```python
from build123d import *

# Parameters (mm, degrees)
F0_W     = 60
F0_H     = 50
F1_DEPTH = 3
F2_W     = 5
F2_H     = 25
F3_DEPTH = 30
F4_R     = 12.49999
F5_R     = 3
F6_DEPTH = 50
F7_R     = 2.5
F8_DEPTH = 25


# Not quite as in the source:
# - a fillet or chamfer is up to 0.001 mm smaller than in the source, because OpenCascade refuses the exact size


with BuildPart() as f1:
    # F0 (on Top) → F1 (new body)
    with BuildSketch(Plane.XY):
        Rectangle(F0_W, F0_H)
    extrude(amount=F1_DEPTH)

    # F2 (on face) → F3 (join)
    with BuildSketch(Plane.XY.offset(3)):
        with Locations((-11.5, 0)):
            Rectangle(F2_W, F2_H)
        with Locations((11.5, 0)):
            Rectangle(F2_W, F2_H)
    extrude(amount=F3_DEPTH)

    # F4 (radius 12.5 in the source; OpenCascade refuses exactly that, so slightly less here)
    f4_edges = [f1.edges().sort_by_distance(p)[0] for p in [
        (-11.5, -12.5, 33),
        (-11.5, 12.5, 33),
        (11.5, 12.5, 33),
        (11.5, -12.5, 33),
    ]]
    fillet(f4_edges, radius=F4_R)

    # F5 (on face) → F6 (cut)
    with BuildSketch(Plane(origin=(-14, 0, 0), x_dir=(0, -1, 0), z_dir=(-1, 0, 0))):
        with Locations((0, 20.5)):
            Circle(F5_R)
    extrude(amount=-F6_DEPTH, mode=Mode.SUBTRACT)

    # F7 (on face) → F8 (cut)
    with BuildSketch(Plane.XY.offset(3)):
        with Locations((-20, -15)):
            Circle(F7_R)
        with Locations((-20, 15)):
            Circle(F7_R)
        with Locations((20, 15)):
            Circle(F7_R)
        with Locations((20, -15)):
            Circle(F7_R)
    extrude(amount=-F8_DEPTH, mode=Mode.SUBTRACT)


solid = f1.part
```
Verification items for the finished model (mm, model axes). A direction names the side the tool comes from. Coordinates: 2 decimals unless noted, no trailing zeros. Loops run counter-clockwise (first coordinate to the right, second up) from the corner with the lowest first, then second, coordinate; pieces in that order, holes last. Notation, with made-up numbers: (-26.5, -5) - (8.5, -5) arc R24 cw to (8.5, 5) - close; hole circle Ø7 at (69, 47.5). An arc over 180 degrees is marked (long way). Put each result on its own line as item: value.
Item 1: Section check D-D (x = -20). Enter the section's corners in (y, z).
Conclusion:
outline: (-25, 0) - (-17.5, 0) - (-17.5, 3) - (-25, 3) - close; (-12.5, 0) - (12.5, 0) - (12.5, 3) - (-12.5, 3) - close; (17.5, 0) - (25, 0) - (25, 3) - (17.5, 3) - close
Item 2: Section check C-C (z = 7). Enter the section's corners in (x, y), then the cut area to 3 significant figures.
Conclusion:
outline: (-14, -12.5) - (-9, -12.5) - (-9, 12.5) - (-14, 12.5) - close; (9, -12.5) - (14, -12.5) - (14, 12.5) - (9, 12.5) - close
area: 250 mm2
Item 3: Set-up check for faces 5 (the face through (11, -12.5, 12)), 6 (the face through (14, 0, 14)), 7 (the face through (9, 0, 14)): record each of +Z, -Z, +X, -X, +Y, -Y from which the full face is reachable in a straight line by a thin tool's end or side.
Conclusion:
face 5: +Z, +X, -X, -Y
face 6: +Z, +X, +Y, -Y
face 7: +Z, +Y, -Y
Item 4: Scan lines: line 1 along Y through (x, z) = (20, 1); line 2 along X through (y, z) = (9.5, 4); line 3 along Z through (x, y) = (10, 0). Record each from-to range of solid material in increasing order.
Conclusion:
line 1: y = -25 to -17.5, -12.5 to 12.5, 17.5 to 25
line 2: x = -14 to -9, 9 to 14
line 3: z = 0 to 17.5, 23.5 to 33
Item 5: Section check A-A (y = 15). Enter the section's corners in (x, z).
Conclusion:
outline: (-30, 0) - (-22.5, 0) - (-22.5, 3) - (-30, 3) - close; (-17.5, 0) - (17.5, 0) - (17.5, 3) - (-17.5, 3) - close; (22.5, 0) - (30, 0) - (30, 3) - (22.5, 3) - close
Item 6: Draft check along Y on faces 1 (the face through (11.535, 8.935, 29.241)), 2 (the face through (-12, -12.5, 12)), 3 (the face through (11.46, 0.65, 17.57)), 4 (the face through (-14, 0, 14)). Enter one of: pulls with the +Y half, pulls with the -Y half, needs draft (parallel to the pull), parting line crosses it, or undercut.
Conclusion:
face 1: pulls with the +Y half
face 2: pulls with the -Y half
face 3: undercut
face 4: needs draft
Item 7: Gauge pin test, flat ends, axial feed: pin 1 Ø8 at (y, z) = (0, 20.5) entering from +X; pin 2 Ø2 at (x, z) = (-9.5, 17.5) entering from +Y; pin 3 Ø5 at (x, y) = (17.5, -15.5) entering from -Z; pin 4 Ø8 at (x, y) = (20, 15) entering from +Z. Record the tip position at first contact, or that the pin passes through.
Conclusion:
pin 1: stops at x = 14
pin 2: stops at y = 12.5
pin 3: stops at z = 0
pin 4: stops at z = 3
